Could you check a few things on this model? Use its own coordinates, in mm. Give positions to 0.01 mm unless a question says otherwise; leave off trailing zeros. Order: outer loops, then holes, each group sorted by start corner. A loop starts at its lowest first (then second) coordinate and runs counter-clockwise, first axis right, second up. Notation, with made-up numbers: M -36.75,84 L -1.75,84 A31 ccw -1.75,110 Z; hole C 58.5,-7.75 d6. An arc over 180 degrees is marked long. Use a Markdown table: item, result. Add a question column.
Item 1: Suppose I cut it at A-A on y = 0. Write out the boundary of the cut face in (x, z), plus the area to 3 significant figures.
Item 2: Suppose I cut it at D-D on y = 96.5. Write out the boundary of the cut face in (x, z).
Item 3: If I drill on L1, parallel to X at y = 35.5, z = 1.6; L2, parallel to X at y = -47, z = 1.2; L3, parallel to Y at x = 3.5, z = 1.5, over which ranges is the centre line in solid material (lowest first)? Write a range as from..to.
Item 4: I'm going to push a flat-ended pin straight in: pin 1 Ø5 at (x, y) = (85.355, -35.355) entering from -Z. Where does the tip first touch, or does it pass through?
Item 5: Suppose I cut it at C-C on z = 0.65. Count the separate pieces of the cut face and the enclosed holes in it, plus the area to 3 significant figures.
Item 6: Suppose I cut it at B-B on x = -20. Write out the boundary of the cut face in (y, z).
Solid Edge part; units mm, degrees
sketch "Sketch1" plane through (0, 0, 0) normal (0, 0, 1) x (1, 0, 0)
  line L0 (-120, -150) -> (120, -150)
  arc A0 (150, -120) -> (120, -150) centre (120, -120) cw
  line L1 (150, -120) -> (150, 120)
  arc A1 (120, 150) -> (150, 120) centre (120, 120) cw
  line L2 (120, 150) -> (-120, 150)
  arc A2 (-120, 150) -> (-150, 120) centre (-120, 120) ccw
  line L3 (-150, 120) -> (-150, -120)
  arc A3 (-150, -120) -> (-120, -150) centre (-120, -120) ccw
  circle A4 centre (50, 0) radius 26.5
  circle A5 centre (-20, 0) radius 20
  circle A6 centre (3.5, 23.5) radius 2.5
  circle A7 centre (-43.5, 23.5) radius 2.5
  circle A8 centre (-43.5, -23.5) radius 2.5
  circle A9 centre (3.5, -23.5) radius 2.5
extrude "Protrusion1" add sketch "Sketch1" along normal blind 4
sketch "Sketch2" plane through (0, 0, 4) normal (0, 0, 1) x (1, 0, 0)
  circle A0 centre (14.645, -35.355) radius 3
  circle A1 centre (85.355, -35.355) radius 3
  circle A2 centre (85.355, 35.355) radius 3
  circle A3 centre (14.645, 35.355) radius 3
extrude "ExtrudedCutout_1" cut sketch "Sketch2" against normal blind 10
sketch "Sketch3" plane through (0, 0, 4) normal (0, 0, 1) x (1, 0, 0)
  circle A0 centre (30.325, 47.5) radius 3.175
  circle A1 centre (69.675, 47.5) radius 3.175
  circle A2 centre (69.675, -47.5) radius 3.175
  circle A3 centre (30.325, -47.5) radius 3.175
extrude "Cutout1" cut sketch "Sketch3" against normal blind 88
sketch "Sketch4" plane through (0, 0, 4) normal (0, 0, 1) x (1, 0, 0)
  circle A0 centre (10, 110) radius 22.3607
extrude "ExtrudedCutout_3" cut sketch "Sketch4" against normal blind 150
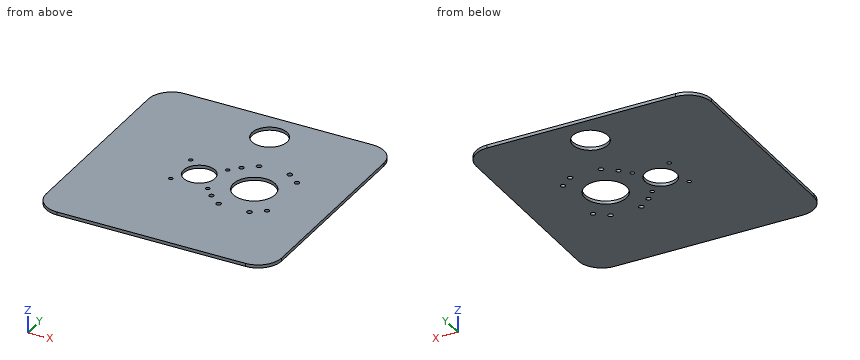
Findings below:
| question | item | result |
|---|---|---|
| 1 | outline | M -150,0 L -40,0 L -40,4 L -150,4 Z; M 0,0 L 23.5,0 L 23.5,4 L 0,4 Z; M 76.5,0 L 150,0 L 150,4 L 76.5,4 Z |
| 1 | area | 828 mm^2 |
| 2 | outline | M -150,0 L -7.83,0 L -7.83,4 L -150,4 Z; M 27.83,0 L 150,0 L 150,4 L 27.83,4 Z |
| 3 | L1 | x = -150..11.65, 17.64..82.36, 88.35..150 |
| 3 | L2 | x = -150..27.19, 33.46..66.54, 72.81..150 |
| 3 | L3 | y = -150..-26, -21..21, 26..88.6, 131.4..150 |
| 4 | pin 1 | passes through |
| 5 | separate pieces | 1 |
| 5 | enclosed holes | 15 |
| 5 | area | 83,900 mm^2 |
| 6 | outline | M -150,0 L -20,0 L -20,4 L -150,4 Z; M 20,0 L 150,0 L 150,4 L 20,4 Z |
